Source: CAD feature listing. Evaluate the final solid. Frame: model axes, mm. A direction names the side the tool comes from. Round coordinates to 2 decimals unless told otherwise and drop trailing zeros. Order: outer loops, then holes, each group sorted by start corner. A loop starts at its lowest first (then second) coordinate and runs counter-clockwise, first axis right, second up. Notation, with made-up numbers: (17.25, 65) -> (52.25, 65) arc R12 cw to (52.25, 78) -> close; hole circle Ø5 at (0.5, 86.5). An arc over 180 degrees is marked (long way). Answer as CSV lines item,"result".
from build123d import *

# Parameters (mm, degrees)
SKETCH1_R           = 3.175
BOSS_EXTRUDE1_DEPTH = 3.175


with BuildPart() as part:
    # Sketch1 → Boss-Extrude1 (new body, symmetric)
    with BuildSketch(Plane(origin=(0, 0, 0), x_dir=(1, 0, 0), z_dir=(0, 1, 0))):
        with BuildLine():
            Line((4.10493597, 8.59506403), (17.575320151, 22.065448212))
            Line((17.575320151, 22.065448212), (19.371371376, 20.269396988))
            Line((19.371371376, 20.269396988), (22.065448212, 22.963473824))
            Line((22.065448212, 22.963473824), (20.269396988, 24.759525048))
            Line((20.269396988, 24.759525048), (22.065448212, 26.555576272))
            Line((22.065448212, 26.555576272), (26.555576272, 22.065448212))
            ThreePointArc((26.555576272, 22.065448212), (22.310576634, -15.991639638), (6.35, -50.8))
            Line((6.35, -50.8), (-6.35, -50.8))
            Line((-6.35, -50.8), (-6.35, -7.099515829))
            ThreePointArc((-6.35, -7.099515829), (-7.92717083, 5.280680604), (4.10493597, 8.59506403))
        make_face()
        Circle(SKETCH1_R, mode=Mode.SUBTRACT)
    extrude(amount=BOSS_EXTRUDE1_DEPTH, both=True)


solid = part.part
1. Mould query, pull axis Z, two halves, no side actions, for faces 1 (the flat face through (18.46, 0.04, -21.18)), 2 (the flat face through (-6.35, 0, 29)), 3 (the cylindrical face through (-8.03, 0.04, -5.12)), 4 (the cylindrical face through (-0.69, -0.04, 3.1)). Classes: released by +Z, released by -Z, zero draft, split by the parting line, or undercut.
Results below:
face 1,"released by -Z"
face 2,"zero draft"
face 3,"split by the parting line"
face 4,"undercut"
2. Section query C-C on z = 0. Return loops of the section in (x, y) (3 decimals), and give its area (3 significant figures).
Results below:
outline,"(-9.525, -3.175) -> (-3.175, -3.175) -> (-3.175, 3.175) -> (-9.525, 3.175) -> close; (3.175, -3.175) -> (25.598, -3.175) -> (25.598, 3.175) -> (3.175, 3.175) -> close"
area,"183 mm2"
3. Section query D-D on x = 11. Return loops of the section in (y, z) (3 decimals), and give its area (3 significant figures).
Results below:
outline,"(-3.175, -15.49) -> (3.175, -15.49) -> (3.175, 43.26) -> (-3.175, 43.26) -> close"
area,"373 mm2"
4. Section query A-A on y = 1.5. Return loops of the section in (x, z) (3 decimals), and give its area (3 significant figures).
Results below:
outline,"(-6.35, 7.1) arc R9.525 ccw to (4.105, -8.595) -> (17.575, -22.065) -> (19.371, -20.269) -> (22.065, -22.963) -> (20.269, -24.76) -> (22.065, -26.556) -> (26.556, -22.065) arc R120.612 ccw to (6.35, 50.8) -> (-6.35, 50.8) -> close; hole circle Ø6.35 at (0, 0)"
area,"1,750 mm2"
5. Section query B-B on x = 0. Return loops of the section in (y, z) (3 decimals), and give its area (3 significant figures).
Results below:
outline,"(-3.175, -9.525) -> (3.175, -9.525) -> (3.175, -3.175) -> (-3.175, -3.175) -> close; (-3.175, 3.175) -> (3.175, 3.175) -> (3.175, 50.8) -> (-3.175, 50.8) -> close"
area,"343 mm2"
6. Reachability of faces 5 (the flat face through (20.7, 0, -21.6)), 6 (the flat face through (24.28, 0.04, -24.34)), 7 (the flat face through (21.18, 0.04, -23.85)) from +Z, -Z, +X, -X, +Y, -Y: full face, straight path, thin tool, end or side. Return the list, or none.
Results below:
face 5,"+Y, -Y"
face 6,"-Z, +X, +Y, -Y"
face 7,"-X, +Y, -Y"
7. Pin query (flat end, axial travel): pin 1 (1 mm diameter, centred on y = 0.5, z = -7, fed in from -X); pin 2 (5.5 mm diameter, centred on x = 0, z = 0, fed in from +Y). Return the tip coordinate at first contact, or that it passes through.
Results below:
pin 1,"x = -6.96"
pin 2,"through"
8. Line query: L1, parallel to Z at x = 0, y = 0.75 (3 decimals); L2, parallel to X at y = -0.5, z = 0 (3 decimals); L3, parallel to X at y = 1, z = -11.5. Output: solid intervals per line, ascending. Write a range as [from, to].
Results below:
L1,"[-9.525, -3.175], [3.175, 50.8]"
L2,"[-9.525, -3.175], [3.175, 25.598]"
L3,"[7.01, 26.6]"
